```python
from build123d import *

# Parameters (mm, degrees)
BOSS_EXTRUDE1_DEPTH = 9
SKETCH2_R           = 1
CUT_EXTRUDE1_DEPTH  = 9


with BuildPart() as part:
    # Sketch1 → Boss-Extrude1 (new body)
    with BuildSketch(Plane(origin=(0, 0, 0), x_dir=(1, 0, 0), z_dir=(0, 1, 0))):
        with BuildLine():
            Line((12, 0), (13.31838565, 0))
            Line((13.31838565, 0), (19, 0))
            Line((19, 0), (19, 2))
            Line((19, 2), (15, 2))
            ThreePointArc((15, 2), (14.292893219, 2.292893219), (14, 3))
            Line((14, 3), (14, 11))
            ThreePointArc((14, 11), (13.707106781, 11.707106781), (13, 12))
            Line((13, 12), (-1, 12))
            ThreePointArc((-1, 12), (-1.707106781, 11.707106781), (-2, 11))
            Line((-2, 11), (-2, 3))
            ThreePointArc((-2, 3), (-2.292893219, 2.292893219), (-3, 2))
            Line((-3, 2), (-7, 2))
            Line((-7, 2), (-7, 0))
            Line((-7, 0), (-0.237668161, 0))
            Line((-0.237668161, 0), (0, 0))
            Line((0, 0), (0, 9))
            ThreePointArc((0, 9), (0.292893219, 9.707106781), (1, 10))
            Line((1, 10), (11, 10))
            ThreePointArc((11, 10), (11.707106781, 9.707106781), (12, 9))
            Line((12, 9), (12, 0))
        make_face()
    extrude(amount=BOSS_EXTRUDE1_DEPTH)

    # Sketch2 → Cut-Extrude1 (cut)
    with BuildSketch(Plane(origin=(0, 0, -2), x_dir=(-1, 0, 0), z_dir=(0, 0, -1))):
        with Locations((-17, 7)):
            Circle(SKETCH2_R)
        with Locations((5, 7)):
            Circle(SKETCH2_R)
        with Locations((-17, 2)):
            Circle(SKETCH2_R)
        with Locations((5, 2)):
            Circle(SKETCH2_R)
    extrude(amount=-CUT_EXTRUDE1_DEPTH, mode=Mode.SUBTRACT)


solid = part.part
```
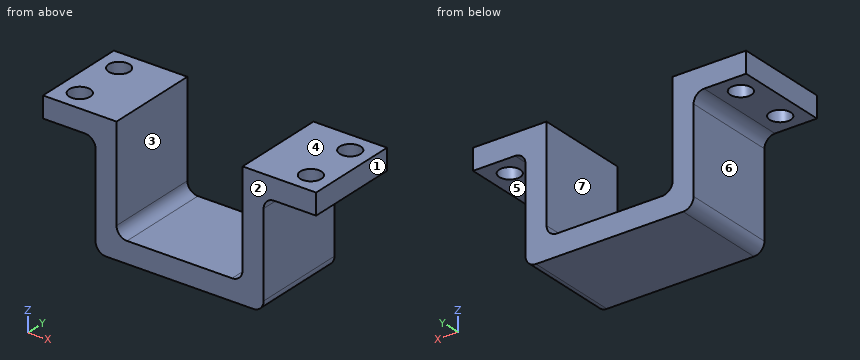
CAD build for the part. Positions are in the model's coordinates, mm. Face numbers are marked on the shaded views. A direction names the side the tool comes from. Round coordinates to 2 decimals unless told otherwise and drop trailing zeros. Write each loop counter-clockwise with the first axis right and the second up, starting at its lowest first coordinate (ties: lowest second). Pieces come first, ordered by that corner, then holes. Notation, with made-up numbers: (-34, 35.5) - (19, 35.5) arc R14 ccw to (19, 45.5) - close; hole circle Ø10 at (-27.5, 41). An arc over 180 degrees is marked (long way). Write item = value, one per line. Start each with the question number.
Q1. Band-saw the part on D-D (z = -9.25). Give the cut face in (x, y), then the cut area to 3 significant figures.
Q2. Probe L1, parallel to Y at x = 17, z = -1.35; L2, parallel to X at y = 3.25, z = -0.5; L3, parallel to X at y = 2, z = -5.5. List the from-to ranges inside material, lowest first. Write a range as from..to.
Q3. Drop flat-ended pins along their axis: pin 1 (5 mm diameter, centred on y = 3, z = -10, fed in from +X); pin 2 (2 mm diameter, centred on x = 16, y = 2.5, fed in from -Z); pin 3 (4 mm diameter, centred on x = 3, y = 7, fed in from +Z). Give the stop position or say it passes through.
Q4. Band-saw the part on B-B (x = -5). Give the cut face in (y, z), then the cut area to 3 significant figures.
Q5. Band-saw the part on A-A (z = -1.5). Give the cut face in (x, y), then the cut area to 3 significant figures.
Q6. Mould opens along X. For the marked faces 1, 2 and 3 say: pulls with the +X half, pulls with the -X half, needs draft (parallel to the pull), parting line crosses it, or undercut.
Q7. Which spindle directions (+Z, -Z, +X, -X, +Y, -Y) get a long thin tool onto all of the face, cutting with end or side? Do the marked faces 4, 5, 6 and 7. Say none if no direction does.
Q8. Band-saw the part on C-C (y = 2). Give the cut face in (x, z).
Answers below:
q1.outline = (-2, 0) - (0.03, 0) - (0.03, 9) - (-2, 9) - close; (11.97, 0) - (14, 0) - (14, 9) - (11.97, 9) - close
q1.area = 36.6 mm2
q2.L1 = 0..1, 3..6, 8..9
q2.L2 = -7..0, 12..19
q2.L3 = -2..0, 12..14
q3.pin_1 = 14
q3.pin_2 = -2
q3.pin_3 = -10
q4.outline = (0, -2) - (1, -2) - (1, 0) - (0, 0) - close; (3, -2) - (6, -2) - (6, 0) - (3, 0) - close; (8, -2) - (9, -2) - (9, 0) - (8, 0) - close
q4.area = 10.0 mm2
q5.outline = (-7, 0) - (0, 0) - (0, 9) - (-7, 9) - close; (12, 0) - (19, 0) - (19, 9) - (12, 9) - close; hole circle Ø2 at (-5, 2); hole circle Ø2 at (-5, 7); hole circle Ø2 at (17, 2); hole circle Ø2 at (17, 7)
q5.area = 113 mm2
q6.face_1 = pulls with the +X half
q6.face_2 = needs draft
q6.face_3 = undercut
q7.face_4 = +Z, +X, -X, +Y, -Y
q7.face_5 = -Z, +X, +Y, -Y
q7.face_6 = -Z, -X, +Y, -Y
q7.face_7 = +Z, +Y, -Y
q8.outline = (-7, -2) - (-6, -2) - (-6, 0) - (-7, 0) - close; (-4, -2) - (-3, -2) arc R1 cw to (-2, -3) - (-2, -11) arc R1 ccw to (-1, -12) - (13, -12) arc R1 ccw to (14, -11) - (14, -3) arc R1 cw to (15, -2) - (16, -2) - (16, 0) - (12, 0) - (12, -9) arc R1 cw to (11, -10) - (1, -10) arc R1 cw to (0, -9) - (0, 0) - (-4, 0) - close; (18, -2) - (19, -2) - (19, 0) - (18, 0) - close
